```python
from build123d import *

# Parameters (mm, degrees)
CUT_EXTRUDE1_DEPTH      = 4.1496001
CUT_EXTRUDE1_DEPTH_BACK = 4.1496001
CUT_EXTRUDE2_DEPTH      = 4.1496001
CUT_EXTRUDE2_DEPTH_BACK = 4.1496001
FILLET2_R               = 0.254
SKETCH7_W               = 1.840958013
SKETCH7_H               = 16.135739168
CUT_EXTRUDE3_DEPTH      = 4.1496001
CUT_EXTRUDE3_DEPTH_BACK = 4.1496001


with BuildPart() as part:
    # Sketch2 → Revolve1 (revolve)
    with BuildSketch(Plane(origin=(0, 0, 0), x_dir=(0, 0, -1), z_dir=(1, 0, 0))):
        with BuildLine():
            Line((-16.5862, 0), (-16.5862, 0.79375))
            Line((-16.5862, 0.79375), (-1.2954, 0.79375))
            ThreePointArc((-1.2954, 0.79375), (-1.001833933, 2.097500262), (-0.1778, 3.1496))
            Line((-0.1778, 3.1496), (0, 3.1496))
            Line((0, 3.1496), (0, 1.5875))
            Line((0, 1.5875), (7.6454, 1.5875))
            Line((7.6454, 1.5875), (7.6454, 1.496709354))
            Line((7.6454, 1.496709354), (7.6454, 0))
            Line((7.6454, 0), (-16.5862, 0))
        make_face()
    revolve(axis=Axis((0, 0, 16.5862), (0, 0, -1)))

    # Sketch3 → Cut-Extrude1 (cut, two sides)
    with BuildSketch(Plane(origin=(0, 0, 0), x_dir=(1, 0, 0), z_dir=(0, 1, 0))) as cut_extrude1_sk:
        Polygon((0, -16.5862), (0.99695, -15.286949465), (0.99695, -17.0942), (-0.99695, -17.0942), (-0.99695, -15.286949465), align=None)
    extrude(amount=CUT_EXTRUDE1_DEPTH, mode=Mode.SUBTRACT)
    extrude(cut_extrude1_sk.sketch, amount=-CUT_EXTRUDE1_DEPTH_BACK, mode=Mode.SUBTRACT)

    # Sketch5 → Cut-Extrude2 (cut, two sides)
    with BuildSketch(Plane(origin=(0, 0, 0), x_dir=(0, 0, -1), z_dir=(1, 0, 0))) as cut_extrude2_sk:
        Polygon((-16.5862, 0), (-15.55176486, 1.11125), (-16.9037, 1.11125), (-16.9037, -1.11125), (-15.55176486, -1.11125), align=None)
    extrude(amount=CUT_EXTRUDE2_DEPTH, mode=Mode.SUBTRACT)
    extrude(cut_extrude2_sk.sketch, amount=-CUT_EXTRUDE2_DEPTH_BACK, mode=Mode.SUBTRACT)

    # Fillet2
    fillet2_edges = [part.edges().sort_by_distance(p)[0] for p in [
        (0, -1.5875, 0),
    ]]
    fillet(fillet2_edges, radius=FILLET2_R)

    # Sketch7 → Cut-Extrude3 (cut, two sides)
    with BuildSketch(Plane(origin=(0, 0, 0), x_dir=(1, 0, 0), z_dir=(0, 1, 0))) as cut_extrude3_sk:
        with Locations((0.126729007, -9.363269584)):
            Rectangle(SKETCH7_W, SKETCH7_H)
    extrude(amount=CUT_EXTRUDE3_DEPTH, mode=Mode.SUBTRACT)
    extrude(cut_extrude3_sk.sketch, amount=-CUT_EXTRUDE3_DEPTH_BACK, mode=Mode.SUBTRACT)


solid = part.part
```
Work out the finished part from the listing and answer in its coordinate system (mm). A direction names the side the tool comes from. Give positions to 0.01 mm unless a question says otherwise; leave off trailing zeros. Loops run counter-clockwise (first coordinate to the right, second up) from the corner with the lowest first, then second, coordinate; pieces in that order, holes last. Notation, with made-up numbers: M -37,-10.5 L -29,-10.5 A24 cw -29,12.5 Z; hole C 38.5,44.5 d7. An arc over 180 degrees is marked long. One line per item, written item: value. Start each with the question number.
1. Find the intervals of material crossed by probe 1 along X at (y, z) = (0, -3); probe 2 along X at (y, z) = (1.25, -4.25); probe 3 along Z at (x, y) = (-1.25, -2.75), in increasing order.
2. Which of the six approach directions +Z, -Z, +X, -X, +Y, -Y give full straight-line access (tool end or side, diameter ignored) to faces 1 (the face through (-2, 0, 0)), 2 (the face through (0, 0, -7.645))?
3. This flat-tipped pin is pushed along its axis until it touches: P1, Ø3, axis at x = -0.5, z = -2.5, coming from the +Y side. Where does it stop, or does it pass through?
4. Find section A-A (z = -4.75). Give the vertices of the cut face in (x, y) (1 decimal), and give its area (3 significant figures).
Reported:
1. probe 1: x = -1.59 to 1.59
1. probe 2: x = -0.98 to 0.98
1. probe 3: z = 0 to 0.33
2. face 1: -Z
2. face 2: -Z, +X, -X, +Y, -Y
3. P1: stops at y = 1.59
4. outline: C 0,0 d3.2
4. area: 7.92 mm²
